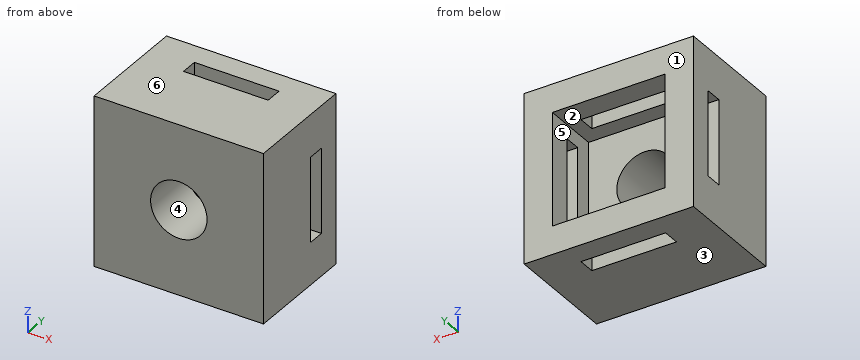
```python
from build123d import *

# Parameters (mm, degrees)
SKETCH1_W           = 15.24
SKETCH1_H           = 15.24
BOSS_EXTRUDE1_DEPTH = 10.16
SKETCH2_R           = 2.54
CUT_EXTRUDE3_DEPTH  = 10.16
SKETCH5_W           = 10.16
SKETCH5_H           = 10.16
CUT_EXTRUDE5_DEPTH  = 5.08
SKETCH7_W           = 7.62
SKETCH7_H           = 1.524
CUT_EXTRUDE6_DEPTH  = 15.24
SKETCH8_W           = 7.62
SKETCH8_H           = 1.524
CUT_EXTRUDE7_DEPTH  = 15.24


with BuildPart() as part:
    # Sketch1 → Boss-Extrude1 (new body)
    with BuildSketch(Plane(origin=(0, 0, 0), x_dir=(1, 0, 0), z_dir=(0, 1, 0))):
        with Locations((7.62, 7.62)):
            Rectangle(SKETCH1_W, SKETCH1_H)
    extrude(amount=BOSS_EXTRUDE1_DEPTH)

    # Sketch2 → Cut-Extrude3 (cut)
    with BuildSketch(Plane(origin=(0, 0, 0), x_dir=(1, 0, 0), z_dir=(0, 1, 0))):
        with Locations((7.62, 7.62)):
            Circle(SKETCH2_R)
    extrude(amount=CUT_EXTRUDE3_DEPTH, mode=Mode.SUBTRACT)

    # Sketch5 → Cut-Extrude5 (cut)
    with BuildSketch(Plane(origin=(0, 10.16, 0), x_dir=(1, 0, 0), z_dir=(0, 1, 0))):
        with Locations((7.62, 7.62)):
            Rectangle(SKETCH5_W, SKETCH5_H)
    extrude(amount=-CUT_EXTRUDE5_DEPTH, mode=Mode.SUBTRACT)

    # Sketch7 → Cut-Extrude6 (cut)
    with BuildSketch(Plane.XY):
        with Locations((7.62, 7.366)):
            Rectangle(SKETCH7_W, SKETCH7_H)
    extrude(amount=-CUT_EXTRUDE6_DEPTH, mode=Mode.SUBTRACT)

    # Sketch8 → Cut-Extrude7 (cut)
    with BuildSketch(Plane(origin=(15.24, 0, 0), x_dir=(0, 0, -1), z_dir=(1, 0, 0))):
        with Locations((7.62, 7.366)):
            Rectangle(SKETCH8_W, SKETCH8_H)
    extrude(amount=-CUT_EXTRUDE7_DEPTH, mode=Mode.SUBTRACT)


solid = part.part
```
Source: CAD feature listing. Evaluate the final solid. Frame: model axes, mm. Face numbers are marked on the shaded views. A direction names the side the tool comes from. Round coordinates to 2 decimals unless told otherwise and drop trailing zeros. Write each loop counter-clockwise with the first axis right and the second up, starting at its lowest first coordinate (ties: lowest second). Pieces come first, ordered by that corner, then holes. Notation, with made-up numbers: M -12,31 L -7,31 A27 cw -7,59 Z; hole C 87,41 d9. An arc over 180 degrees is marked long. Use CSV: the item, a comma, the result in double quotes. Start each with the question number.
Q1. Access query for the marked faces 1 and 2. Directions: +Z, -Z, +X, -X, +Y, -Y. A direction counts if a zero-diameter tool reaches every point of the face in a straight line with its end or side. Return the directions, or none.
Q2. Cut plane D-D on x = 7.62. Output: boundary loops of the cut face in (y, z).
Q3. Cut plane B-B on x = 4.5. Output: boundary loops of the cut face in (y, z).
Q4. Pull-direction query (Z, two-part tool) for the marked faces 3, 4, 5 and 6; classes: +Z half, -Z half, draft (parallel to the pull), parting line (faces both ways), or undercut.
Q5. Line query: line 1 (Z direction, x = 10.5, y = 6.5); line 2 (Z direction, x = 7.62, y = 4); line 3 (Y direction, x = 4, z = -14.25). Output: solid intervals per line, ascending. Write a range as from..to.
Q6. Cut plane A-A on z = -10.75. Output: boundary loops of the cut face in (x, y), plus the area to 3 significant figures.
Q7. Cut plane C-C on y = 7. Output: boundary loops of the cut face in (x, z), plus the area to 3 significant figures.
Q8. First-contact query: P1, Ø5, axis at x = 5.5, z = -6, coming from the +Y side. Flat tip, straight axial feed; report the tip coordinate or a pass-through.
Results found:
1,face 1,"+Z, -Z, +X, -X, +Y"
1,face 2,"+Y"
2,outline,"M 0,-15.24 L 6.6,-15.24 L 6.6,-12.7 L 5.08,-12.7 L 5.08,-10.16 L 0,-10.16 Z; M 0,-5.08 L 5.08,-5.08 L 5.08,-2.54 L 6.6,-2.54 L 6.6,0 L 0,0 Z; M 8.13,-15.24 L 10.16,-15.24 L 10.16,-12.7 L 8.13,-12.7 Z; M 8.13,-2.54 L 10.16,-2.54 L 10.16,0 L 8.13,0 Z"
3,outline,"M 0,-15.24 L 6.6,-15.24 L 6.6,-12.7 L 5.08,-12.7 L 5.08,-2.54 L 6.6,-2.54 L 6.6,0 L 0,0 Z; M 8.13,-15.24 L 10.16,-15.24 L 10.16,-12.7 L 8.13,-12.7 Z; M 8.13,-2.54 L 10.16,-2.54 L 10.16,0 L 8.13,0 Z"
4,face 3,"-Z half"
4,face 4,"undercut"
4,face 5,"undercut"
4,face 6,"+Z half"
5,line 1,"-15.24..-12.7, -2.54..0"
5,line 2,"-15.24..-10.16, -5.08..0"
5,line 3,"0..6.6, 8.13..10.16"
6,outline,"M 0,0 L 15.24,0 L 15.24,6.6 L 12.7,6.6 L 12.7,5.08 L 2.54,5.08 L 2.54,6.6 L 0,6.6 Z; M 0,8.13 L 2.54,8.13 L 2.54,10.16 L 0,10.16 Z; M 12.7,8.13 L 15.24,8.13 L 15.24,10.16 L 12.7,10.16 Z"
6,area,"95.5 mm^2"
7,outline,"M 0,-15.24 L 3.81,-15.24 L 3.81,-12.7 L 2.54,-12.7 L 2.54,-11.43 L 0,-11.43 Z; M 0,-3.81 L 2.54,-3.81 L 2.54,-2.54 L 3.81,-2.54 L 3.81,0 L 0,0 Z; M 11.43,-15.24 L 15.24,-15.24 L 15.24,-11.43 L 12.7,-11.43 L 12.7,-12.7 L 11.43,-12.7 Z; M 11.43,-2.54 L 12.7,-2.54 L 12.7,-3.81 L 15.24,-3.81 L 15.24,0 L 11.43,0 Z"
7,area,"51.6 mm^2"
8,P1,"y = 5.08"
